The model under review builds one solid part; all positions refer to its coordinate system, in mm. A direction names the side the tool comes from. Coordinates: 2 decimals unless noted, no trailing zeros. Order: outer loops, then holes, each group sorted by start corner. A loop starts at its lowest first (then second) coordinate and runs counter-clockwise, first axis right, second up. Notation, with made-up numbers: (23.5, 26) -> (27.5, 26) arc R15 ccw to (27.5, 40) -> close; hole circle Ø5 at (-34, 23). An arc over 180 degrees is marked (long way). Answer as CSV lines item,"result". Start each with the question number.
from build123d import *

# Parameters (mm, degrees)
SKETCH1_R               = 25.4
BOSS_EXTRUDE1_DEPTH     = 152.4
SKETCH2_R               = 9.525
BOSS_EXTRUDE2_DEPTH     = 25.4
SKETCH3_R               = 6.35
CUT_EXTRUDE1_DEPTH      = 100.33
CUT_EXTRUDE2_DEPTH      = 182.392282085
CUT_EXTRUDE2_DEPTH_BACK = 182.392282085
SKETCH4_W               = 19.05
SKETCH4_H               = 3.175
CUT_EXTRUDE3_DEPTH      = 183.389864028
CUT_EXTRUDE3_DEPTH_BACK = 183.389864028
SKETCH5_R               = 4.7625


with BuildPart() as part:
    # Sketch1 → Boss-Extrude1 (new body)
    with BuildSketch(Plane.XY):
        with Locations(Location((0, 0, 0), (0, 0, 180))):
            Circle(SKETCH1_R)
    extrude(amount=BOSS_EXTRUDE1_DEPTH)

    # Sketch2 → Boss-Extrude2 (add)
    with BuildSketch(Plane.XY.offset(152.4)):
        Circle(SKETCH2_R)
    extrude(amount=BOSS_EXTRUDE2_DEPTH)

    # Sketch3 → Cut-Extrude1 (cut)
    with BuildSketch(Plane(origin=(0, 0, 0), x_dir=(-1, 0, 0), z_dir=(0, 0, -1))):
        Circle(SKETCH3_R)
    extrude(amount=-CUT_EXTRUDE1_DEPTH, mode=Mode.SUBTRACT)

    # Sketch4 → Cut-Extrude2 (cut, two sides: drawn at the far end of the back side and taken through both)
    with BuildSketch(Plane(origin=(0, 0, 0), x_dir=(0, 0, -1), z_dir=(1, 0, 0)).offset(-CUT_EXTRUDE2_DEPTH_BACK)):
        with Locations((-168.275, 7.9375)):
            Rectangle(SKETCH4_W, SKETCH4_H)
        with Locations((-168.275, -7.9375)):
            Rectangle(SKETCH4_W, SKETCH4_H)
    extrude(amount=CUT_EXTRUDE2_DEPTH + CUT_EXTRUDE2_DEPTH_BACK, mode=Mode.SUBTRACT)

    # Sketch5 → Cut-Extrude3 (cut, two sides: drawn at the far end of the back side and taken through both)
    with BuildSketch(Plane.XZ.offset(6.35).offset(-CUT_EXTRUDE3_DEPTH_BACK)):
        with Locations(Location((0, 168.275, 0), (0, 0, 270))):
            Circle(SKETCH5_R)
    extrude(amount=CUT_EXTRUDE3_DEPTH + CUT_EXTRUDE3_DEPTH_BACK, mode=Mode.SUBTRACT)


solid = part.part
1) Wall thickness on L1, parallel to Y at x = 0, z = 42; L2, parallel to Z at x = 0, y = -2.75; L3, parallel to Z at x = 11, y = 9.5: over which ranges is each line inside the solid? List them lowest first. Write a range as [from, to].
2) Insertion check: pin 1 Ø6 at (x, z) = (-4.5, 93.5) entering from +Y; pin 2 Ø5 at (y, z) = (-13, 128) entering from +X; pin 3 Ø12 at (x, y) = (16.5, -9) entering from +Z; pin 4 Ø7.5 at (x, z) = (0, 168.275) entering from +Y. Each pin has a flat end and moves straight along its axis. Give the tip position at first contact, or say it passes through.
3) Tool access review of faces 5 (the face through (-11.721, 22.534, 75.133)), 6 (the face through (-5, 6.35, 168)), 7 (the face through (-11, 0, 152.4)), 8 (the face through (0, -8, 158.75)), 9 (the face through (-5, 5, 0)): name each direction out of +Z, -Z, +X, -X, +Y, -Y from which nothing blocks a thin tool from reaching the whole face with its end or side.
4) Mouldability with a two-part tool opening along Z and no side actions: class faces 1 (the face through (0, 8, 158.75)), 2 (the face through (0, 0, 100.33)), 3 (the face through (0.209, 0.089, 173.033)), 4 (the face through (1.38, -6.2, 49.46)) as released by +Z, released by -Z, zero draft, split by the parting line, or undercut.
5) Consider section D-D (z = 148.5). Give the boundary of the cut face in (x, y).
6) Consider section C-C (z = 49.5). Give the boundary of the cut face in (x, y).
Result:
1,L1,"[-25.4, -6.35], [6.35, 25.4]"
1,L2,"[100.33, 163.51], [173.04, 177.8]"
1,L3,"[0, 152.4]"
2,pin 1,"y = 25.36"
2,pin 2,"x = 23.13"
2,pin 3,"z = 152.4"
2,pin 4,"through"
3,face 5,"+Z, -Z"
3,face 6,"+Z, +X, -X, +Y"
3,face 7,"+Z"
3,face 8,"+Z, +X, -X, -Y"
3,face 9,"-Z, +X, -X, +Y, -Y"
4,face 1,"released by +Z"
4,face 2,"released by -Z"
4,face 3,"undercut"
4,face 4,"zero draft"
5,outline,"circle Ø50.8 at (0, 0)"
6,outline,"circle Ø50.8 at (0, 0); hole circle Ø12.7 at (0, 0)"
